```python
from build123d import *

# Parameters (mm, degrees)
SKETCH1_R              = 5
SKETCH1_R_2            = 2.1
BOSS_EXTRUDE1_DEPTH    = 8
SKETCH2_R              = 5
SKETCH2_R_2            = 2
BOSS_EXTRUDE2_DEPTH    = 8
M3_TAPPED_HOLE2_REACH  = 21.519
M3_TAPPED_HOLE2_BORE_R = 1.25


with BuildPart() as part:
    # Sketch1 → Boss-Extrude1 (new body)
    with BuildSketch(Plane(origin=(0, 0, 0), x_dir=(1, 0, 0), z_dir=(0, 1, 0))):
        with Locations(Location((0, 0, 0), (0, 0, 270))):
            Circle(SKETCH1_R)
        with Locations(Location((0, 0, 0), (0, 0, 270))):
            Circle(SKETCH1_R_2, mode=Mode.SUBTRACT)
    extrude(amount=BOSS_EXTRUDE1_DEPTH)

    # Sketch2 → Boss-Extrude2 (add)
    with BuildSketch(Plane(origin=(0, 8, 0), x_dir=(1, 0, 0), z_dir=(0, 1, 0))):
        with Locations(Location((0, 0, 0), (0, 0, 270))):
            Circle(SKETCH2_R)
        with Locations(Location((0, 0, 0), (0, 0, 270))):
            Circle(SKETCH2_R_2, mode=Mode.SUBTRACT)
    extrude(amount=BOSS_EXTRUDE2_DEPTH)

    # M3 Tapped Hole2 bore → M3 Tapped Hole2 (cut, up to next)
    with BuildSketch(Plane.ZY.offset(5), mode=Mode.PRIVATE) as m3_tapped_hole2_sk1:
        with Locations((0, 12.5)):
            Circle(M3_TAPPED_HOLE2_BORE_R)
    m3_tapped_hole2_tool1 = extrude(m3_tapped_hole2_sk1.sketch, amount=-M3_TAPPED_HOLE2_REACH, mode=Mode.PRIVATE) & part.part
    # M3 Tapped Hole2 bore → M3 Tapped Hole2 (cut, up to next)
    with BuildSketch(Plane.ZY.offset(5), mode=Mode.PRIVATE) as m3_tapped_hole2_sk2:
        with Locations((0, 3.5)):
            Circle(M3_TAPPED_HOLE2_BORE_R)
    m3_tapped_hole2_tool2 = extrude(m3_tapped_hole2_sk2.sketch, amount=-M3_TAPPED_HOLE2_REACH, mode=Mode.PRIVATE) & part.part
    add(m3_tapped_hole2_tool1.solids().sort_by_distance((-5, 12.5, 0))[0], mode=Mode.SUBTRACT)
    add(m3_tapped_hole2_tool2.solids().sort_by_distance((-5, 3.5, 0))[0], mode=Mode.SUBTRACT)


solid = part.part
```
CAD build for the part. Positions are in the model's coordinates, mm. A direction names the side the tool comes from. Give positions to 0.01 mm unless a question says otherwise; leave off trailing zeros. Order: outer loops, then holes, each group sorted by start corner. A loop starts at its lowest first (then second) coordinate and runs counter-clockwise, first axis right, second up.
(1) Mould opens along X. For faces 1 (the cylindrical face through (2, 12, 0)), 2 (the cylindrical face through (-4.88, 7.89, -1.08)), 3 (the flat face through (-1, 0, 2.2)) say: released by +X, released by -X, zero draft, split by the parting line, or undercut.
(2) Flat gauge pins, fed straight in: pin 1 (3.5 mm diameter, centred on x = 0, z = 0, fed in from -Y); pin 2 (2 mm diameter, centred on y = 3.5, z = 0, fed in from -X); pin 3 (1.5 mm diameter, centred on x = -2, y = 3, fed in from +Z). Where does each tip first touch, or does it go through?
(3) Tool access for faces 4 (the cylindrical face through (-3.3, 12.55, -1.25)), 5 (the cylindrical face through (2.082, 3.944, -0.273)), 6 (the flat face through (0.1, 16, 2.2)): list every direction of +Z, -Z, +X, -X, +Y, -Y with a clear straight run to the whole face (end or side of a thin tool).
(4) Saw through at D-D, the plane y = 1.75. Give the cut face in (x, z), then the cut area to 3 significant figures.
(5) Saw through at A-A, the plane x = 0. Give the cut face in (y, z).
(6) Saw through at B-B, the plane z = 0. Give the cut face in (x, y), then the cut area to 4 significant figures.
(7) Drill centre lines: L1, parallel to Y at x = -3.85, z = 0; L2, parallel to X at y = 2, z = 0; L3, parallel to Z at x = -3.15, y = 3.5. Where is each one in solid material? Low to high.
(8) Saw through at C-C, the plane x = -2.75. Give the cut face in (y, z).
Results found:
1. face 1: undercut
1. face 2: split by the parting line
1. face 3: zero draft
2. pin 1: passes through
2. pin 2: stops at x = 1.85
2. pin 3: stops at z = 4.84
3. face 4: -X
3. face 5: -Y
3. face 6: +Z, -Z, +X, -X, +Y
4. outline: circle Ø10 at (0, 0); hole circle Ø4.2 at (0, 0)
4. area: 64.7 mm2
5. outline: (0, -5) - (16, -5) - (16, -2) - (8, -2) - (8, -2.1) - (0, -2.1) - close; (0, 2.1) - (8, 2.1) - (8, 2) - (16, 2) - (16, 5) - (0, 5) - close
6. outline: (-5, 0) - (-2.1, 0) - (-2.1, 2.25) - (-5, 2.25) - close; (-5, 4.75) - (-2.1, 4.75) - (-2.1, 8) - (-2, 8) - (-2, 11.25) - (-5, 11.25) - close; (-5, 13.75) - (-2, 13.75) - (-2, 16) - (-5, 16) - close; (2, 8) - (2.1, 8) - (2.1, 0) - (5, 0) - (5, 16) - (2, 16) - close
6. area: 79.65 mm2
7. L1: y = 0 to 2.25, 4.75 to 11.25, 13.75 to 16
7. L2: x = -5 to -2.1, 2.1 to 5
7. L3: z = -3.88 to -1.25, 1.25 to 3.88
8. outline: (0, -4.18) - (16, -4.18) - (16, 4.18) - (0, 4.18) - close; hole circle Ø2.5 at (3.5, 0); hole circle Ø2.5 at (12.5, 0)
